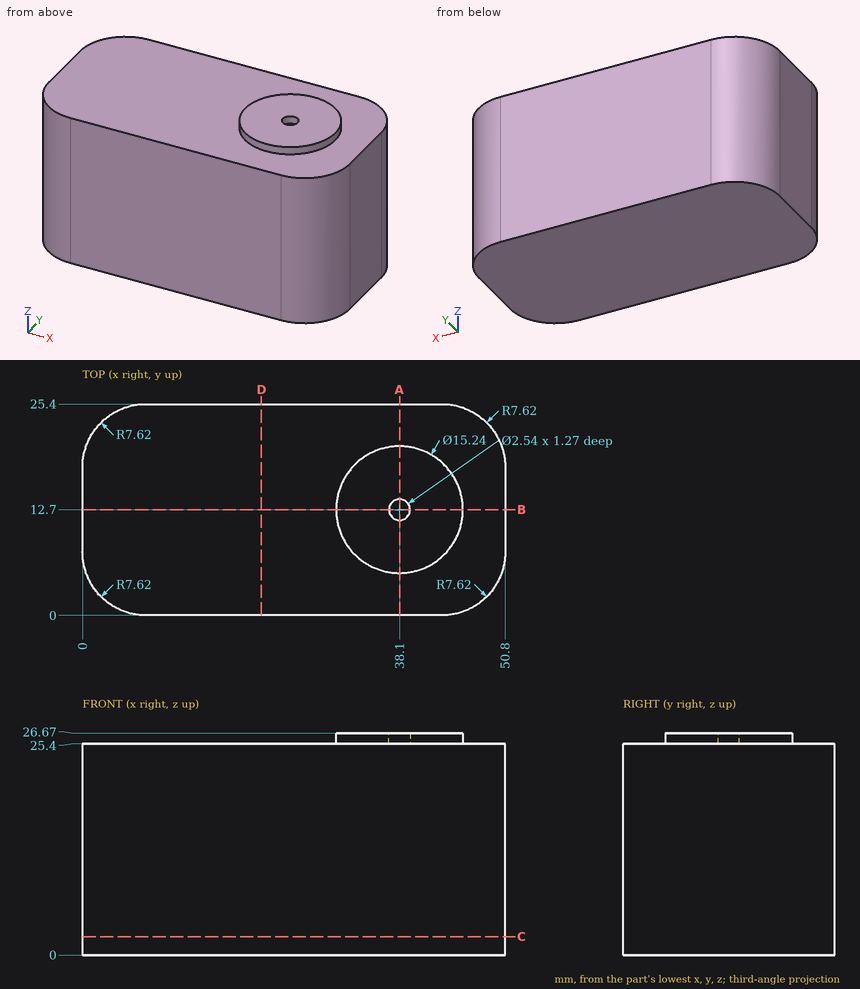
Here's the drawing with two shaded views (mm, measured from the low corner). I have some questions. Give positions to 0.01 mm unless a question says otherwise; leave off trailing zeros. Order: outer loops, then holes, each group sorted by start corner. A loop starts at its lowest first (then second) coordinate and runs counter-clockwise, first axis right, second up. Notation, with made-up numbers: (45, 85.25) -> (88, 85.25) arc R14 cw to (88, 106.25) -> close; hole circle Ø11 at (-10, -20). An arc over 180 degrees is marked (long way). Use a Markdown table: item, result. Add a question column.
Item 1: Imagine slicing it at C-C on z = 2.25. Please give me the cut outline in (x, y).
Item 2: Imagine slicing it at B-B on y = 12.7. Please give me the cut outline in (x, z), plus the area to 3 significant figures.
Item 3: Imagine slicing it at D-D on x = 21.5. Please give me the cut outline in (y, z).
Item 4: I need wall thicknesses on line 1 (Y direction, x = 38.1, z = 26); line 2 (Z direction, x = 13.5, y = 1.75); line 3 (X direction, y = 7.5, z = 18). Which ranges of each line are inside material? Lowest first, please.
Item 5: Imagine slicing it at A-A on x = 38.1. Please give me the cut outline in (y, z).
Data:
| question | item | result |
|---|---|---|
| 1 | outline | (0, 7.62) arc R7.62 ccw to (7.62, 0) -> (43.18, 0) arc R7.62 ccw to (50.8, 7.62) -> (50.8, 17.78) arc R7.62 ccw to (43.18, 25.4) -> (7.62, 25.4) arc R7.62 ccw to (0, 17.78) -> close |
| 2 | outline | (0, 0) -> (50.8, 0) -> (50.8, 25.4) -> (45.72, 25.4) -> (45.72, 26.67) -> (39.37, 26.67) -> (39.37, 25.4) -> (36.83, 25.4) -> (36.83, 26.67) -> (30.48, 26.67) -> (30.48, 25.4) -> (0, 25.4) -> close |
| 2 | area | 1,310 mm² |
| 3 | outline | (0, 0) -> (25.4, 0) -> (25.4, 25.4) -> (0, 25.4) -> close |
| 4 | line 1 | y = 5.08 to 11.43, 13.97 to 20.32 |
| 4 | line 2 | z = 0 to 25.4 |
| 4 | line 3 | x = 0 to 50.8 |
| 5 | outline | (0, 0) -> (25.4, 0) -> (25.4, 25.4) -> (20.32, 25.4) -> (20.32, 26.67) -> (13.97, 26.67) -> (13.97, 25.4) -> (11.43, 25.4) -> (11.43, 26.67) -> (5.08, 26.67) -> (5.08, 25.4) -> (0, 25.4) -> close |
